Geometry check sheet. Reference: the model listing, model coordinates, mm. Face numbers are marked on the shaded views. Coordinates: 2 decimals unless noted, no trailing zeros. Loops run counter-clockwise (first coordinate to the right, second up) from the corner with the lowest first, then second, coordinate; pieces in that order, holes last.
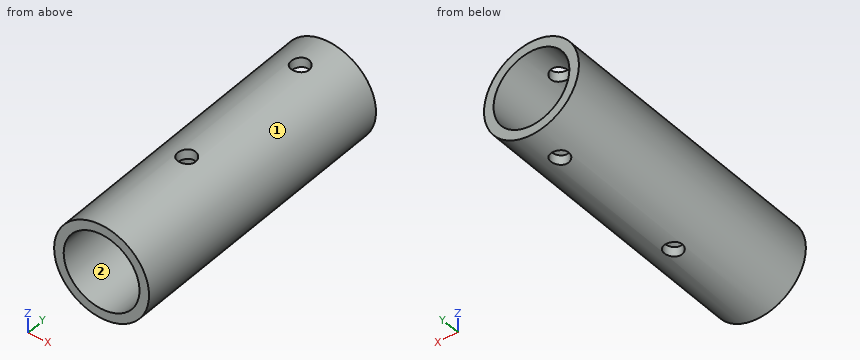
Autodesk Inventor part; units mm, degrees
ref_plane "YZ Plane" through (0, 0, 0) normal (1, 0, 0) x (0, 1, 0)
ref_plane "XZ Plane" through (0, 0, 0) normal (0, 1, 0) x (-1, 0, 0)
ref_plane "XY Plane" through (0, 0, 0) normal (0, 0, 1) x (1, 0, 0)
sketch "Sketch1" plane through (0, 0, 0) normal (0, 1, 0) x (-1, 0, 0)
  circle A0 centre (0, 0) radius 16.7005
  circle A1 centre (0, 0) radius 13.335
  dimension "d0" = 33.401
  dimension "d1" = 26.67
extrude "Extrusion1" add sketch "Sketch1" along normal mid plane 101.6
sketch "Sketch3" plane through (0, 0, 0) normal (0, 0, 1) x (1, 0, 0)
  circle A0 centre (0, 38.1) radius 3.175
  circle A1 centre (0, -12.7) radius 3.175
  line L0 (16.7005, 50.8) -> (-16.7005, 50.8)
  point P0 (0, 0)
  dimension "d10" = 12.7
  dimension "d12" = 6.35
  dimension "d15" = 50.8
extrude "Extrusion3" cut sketch "Sketch3" against normal through all both and the other way through all
properties part number "FE-130-003 Insert" material "Aluminum 6061"
1) Section check B-B on x = 0. Record the cut outline in (y, z) (1 decimal), and give its area (3 significant figures).
Data:
outline: (-50.8, -16.7) - (-15.9, -16.7) - (-15.9, -13.3) - (-50.8, -13.3) - close; (-50.8, 13.3) - (-15.9, 13.3) - (-15.9, 16.7) - (-50.8, 16.7) - close; (-9.5, -16.7) - (34.9, -16.7) - (34.9, -13.3) - (-9.5, -13.3) - close; (-9.5, 13.3) - (34.9, 13.3) - (34.9, 16.7) - (-9.5, 16.7) - close; (41.3, -16.7) - (50.8, -16.7) - (50.8, -13.3) - (41.3, -13.3) - close; (41.3, 13.3) - (50.8, 13.3) - (50.8, 16.7) - (41.3, 16.7) - close
area: 598 mm2
2) Mould release check, pull along Z, two halves, no side actions. Record for the marked faces 1 and 2: +Z half, -Z half, draft (parallel to the pull), parting line (faces both ways), or undercut.
Data:
face 1: parting line
face 2: undercut
3) Section check A-A on z = 0. Record the cut outline in (x, y) (1 decimal).
Data:
outline: (-16.7, -50.8) - (-13.3, -50.8) - (-13.3, 50.8) - (-16.7, 50.8) - close; (13.3, -50.8) - (16.7, -50.8) - (16.7, 50.8) - (13.3, 50.8) - close
4) Depth check by flat-ended pin: pin 1 (6 mm diameter, centred on y = 40.5, z = -8, fed in from -X); pin 2 (1 mm diameter, centred on y = 22.5, z = 9.5, fed in from +X); pin 3 (8 mm diameter, centred on x = 10.5, y = -24.5, fed in from +Z). Enter the tip coordinate at first touch or a pass-through.
Data:
pin 1: stops at x = -15.93
pin 2: stops at x = 14.07
pin 3: stops at z = 15.38
5) Section check C-C on y = 38.1. Record the cut outline in (x, z) (1 decimal).
Data:
outline: (-3.2, -16.4) - (-3.2, -13) arc R13.3 cw to (-3.2, 13) - (-3.2, 16.4) arc R16.7 ccw to start; (3.2, -16.4) arc R16.7 ccw to (3.2, 16.4) - (3.2, 13) arc R13.3 cw to (3.2, -13) - close
6) Material ranges on probe 1 along Y at (x, z) = (0, -15.85) (3 decimals); probe 2 along X at (y, z) = (-37, -4.5); probe 3 along Z at (x, y) = (8, -15.5), recorded low to high.
Data:
probe 1: y = -50.8 to -15.875, -9.525 to 34.925, 41.275 to 50.8
probe 2: x = -16.08 to -12.55, 12.55 to 16.08
probe 3: z = -14.66 to -10.67, 10.67 to 14.66
